Geometry: final body of the model. Coordinates: model frame, mm. A direction names the side the tool comes from. Round coordinates to 2 decimals unless told otherwise and drop trailing zeros. Order: outer loops, then holes, each group sorted by start corner. A loop starts at its lowest first (then second) coordinate and runs counter-clockwise, first axis right, second up. Notation, with made-up numbers: M 75,14.25 L 116,14.25 A25 cw 116,37.25 Z; hole C 14,12 d4. An arc over 180 degrees is marked long. Return JSON: item names as keys, results as strings. Group by question number.
Q1. Cut plane B-B on y = 2.5. Output: boundary loops of the cut face in (x, z) (3 decimals), and give its area (3 significant figures).
Q2. Contact query for flat-ended pins moving along their axis: pin 1 (3 mm diameter, centred on y = 6.5, z = 11, fed in from -X); pin 2 (3.5 mm diameter, centred on x = -1, z = -1.5, fed in from -Y). Output: stop coordinate, or through.
Q3. Mould query, pull axis X, two halves, no side actions, for faces 4 (the face through (-2, 5, 57.15)), 5 (the face through (125.346, 7.915, 0.831)), 6 (the face through (-125.346, 7.915, -0.831)), 7 (the face through (0, 3, -5.715)). Classes: released by +X, released by -X, zero draft, split by the parting line, or undercut.
Q4. Ray query, probe 1 along Z at (x, y) = (0, 8.4); probe 2 along X at (y, z) = (7.7, 0); probe 3 along X at (y, z) = (5.5, 20). Return the intervals inside material, ascending.
Q5. Cut plane C-C on z = -39. Output: boundary loops of the cut face in (x, y) (3 decimals), and give its area (3 significant figures).
Q6. Access query for faces 1 (the face through (128, 6.35, -1)), 2 (the face through (2.8, 6.35, 2.5)), 3 (the face through (-128, 6.35, -1)). Directions: +Z, -Z, +X, -X, +Y, -Y. A direction counts if a zero-diameter tool reaches every point of the face in a straight line with its end or side. Return the directions, or none.
Q7. Cut plane D-D on z = 14. Output: boundary loops of the cut face in (x, y) (3 decimals), and give its area (3 significant figures).
```python
from build123d import *

# Parameters (mm, degrees)
BOSS_EXTRUDE1_DEPTH = 9.525
BOSS_EXTRUDE2_DEPTH = 6.35
BOSS_EXTRUDE3_START = 6.35
SKETCH1_4_R         = 3.4925
BOSS_EXTRUDE3_DEPTH = 3.175


with BuildPart() as part:
    # Sketch1 → Boss-Extrude1 (new body)
    with BuildSketch(Plane(origin=(0, 0, 0), x_dir=(1, 0, 0), z_dir=(0, 1, 0))):
        with BuildLine():
            Line((111.562759472, 57.15), (-111.562759472, 57.15))
            ThreePointArc((-111.562759472, 57.15), (-125.349, 0), (-111.562759472, -57.15))
            Line((-111.562759472, -57.15), (111.562759472, -57.15))
            ThreePointArc((111.562759472, -57.15), (125.349, 0), (111.562759472, 57.15))
        make_face()
        Polygon((-3.299556788, -5.715), (-6.599113577, 0), (-3.299556788, 5.715), (3.299556788, 5.715), (6.599113577, 0), (3.299556788, -5.715), align=None, mode=Mode.SUBTRACT)
    extrude(amount=BOSS_EXTRUDE1_DEPTH)

    # Sketch1_3 → Boss-Extrude2 (add)
    with BuildSketch(Plane(origin=(0, 0, 0), x_dir=(1, 0, 0), z_dir=(0, 1, 0))):
        with BuildLine():
            Line((125.663852802, 57.15), (111.562759472, 57.15))
            ThreePointArc((111.562759472, 57.15), (125.349, 0), (111.562759472, -57.15))
            Line((111.562759472, -57.15), (125.663852802, -57.15))
            ThreePointArc((125.663852802, -57.15), (138.049, 0), (125.663852802, 57.15))
        make_face()
        with BuildLine():
            Line((-111.562759472, 57.15), (-125.663852802, 57.15))
            ThreePointArc((-125.663852802, 57.15), (-138.049, 0), (-125.663852802, -57.15))
            Line((-125.663852802, -57.15), (-111.562759472, -57.15))
            ThreePointArc((-111.562759472, -57.15), (-125.349, 0), (-111.562759472, 57.15))
        make_face()
    extrude(amount=BOSS_EXTRUDE2_DEPTH)

    # Sketch1_4 → Boss-Extrude3 (add)
    with BuildSketch(Plane(origin=(0, 0, 0), x_dir=(1, 0, 0), z_dir=(0, 1, 0)).offset(BOSS_EXTRUDE3_START)):
        Polygon((3.299556788, 5.715), (-3.299556788, 5.715), (-6.599113577, 0), (-3.299556788, -5.715), (3.299556788, -5.715), (6.599113577, 0), align=None)
        Circle(SKETCH1_4_R, mode=Mode.SUBTRACT)
    extrude(amount=BOSS_EXTRUDE3_DEPTH)


solid = part.part
```
Result sheet:
{
 "1": {"outline": "M -125.664,-57.15 L 125.664,-57.15 A138.049 ccw 125.664,57.15 L -125.664,57.15 A138.049 ccw Z; hole M -6.599,0 L -3.3,-5.715 L 3.3,-5.715 L 6.599,0 L 3.3,5.715 L -3.3,5.715 Z", "area": "30,500 mm²"},
 "2": {"pin 1": "stops at x = -137.72", "pin 2": "stops at y = 6.35"},
 "3": {"face 4": "zero draft", "face 5": "released by +X", "face 6": "released by -X", "face 7": "undercut"},
 "4": {"probe 1": "z = -57.15 to -3.49, 3.49 to 57.15", "probe 2": "x = -125.35 to -3.49, 3.49 to 125.35", "probe 3": "x = -136.59 to 136.59"},
 "5": {"outline": "M -132.426,0 L 132.426,0 L 132.426,6.35 L 119.128,6.35 L 119.128,9.525 L -119.128,9.525 L -119.128,6.35 L -132.426,6.35 Z", "area": "2,440 mm²"},
 "6": {"face 1": "+X, +Y", "face 2": "-Y", "face 3": "-X, +Y"},
 "7": {"outline": "M -137.337,0 L 137.337,0 L 137.337,6.35 L 124.565,6.35 L 124.565,9.525 L -124.565,9.525 L -124.565,6.35 L -137.337,6.35 Z", "area": "2,540 mm²"}
}
